Read the model definition and answer for the solid it produces. Units are mm, in the model's axes. A direction names the side the tool comes from. Give positions to 0.01 mm unless a question says otherwise; leave off trailing zeros. Write each loop counter-clockwise with the first axis right and the second up, starting at its lowest first coordinate (ties: lowest second). Pieces come first, ordered by that corner, then holes. Notation, with made-up numbers: (19, 89.25) - (42, 89.25) arc R28 ccw to (42, 110.25) - close; hole circle Ø8 at (8.5, -35.75). An arc over 180 degrees is marked (long way). Use CSV: the item, a comma, the result in double quotes. Start each with the question number.
from build123d import *

# Parameters (mm, degrees)
SKETCH2_OUTSIDE_W       = 53.436
SKETCH2_OUTSIDE_H       = 53.436
CUT_EXTRUDE1_DEPTH      = 8.5
CHAMFER1_SIZE           = 1.754
SKETCH5_W               = 1.79
SKETCH5_H               = 3.988
CUT_EXTRUDE2_DEPTH      = 19
CUT_EXTRUDE2_DEPTH_BACK = 19
SKETCH6_W               = 1.075
SKETCH6_H               = 5.994
CUT_EXTRUDE3_DEPTH      = 19
CUT_EXTRUDE3_DEPTH_BACK = 19


with BuildPart() as part:
    # Sketch1 → Revolve1 (revolve)
    with BuildSketch(Plane.XY, mode=Mode.PRIVATE) as revolve1_sk:
        Polygon((-17.125, 0), (-17, 0), (-17, -2.75), (0, -2.75), (0, 55.25), (-11.75, 55.25), (-18, 53.575317547), (-18, 49.125), (-16.875, 48), (-16.875, 46.5), (-17.925, 45.45), (-17.925, 7.45), (-17.125, 6.65), align=None)
    revolve(revolve1_sk.sketch.rotate(Axis((0, 0, 0), (0, -1, 0)), 270), axis=Axis((0, 0, 0), (0, -1, 0)))  # turned: the seam where the file's is

    # Sketch2 outside → Cut-Extrude1 (cut)
    with BuildSketch(Plane(origin=(0, 55.25, 0), x_dir=(1, 0, 0), z_dir=(0, 1, 0))):
        Rectangle(SKETCH2_OUTSIDE_W, SKETCH2_OUTSIDE_H)
        Polygon((0, 18.429020593), (-15.96, 9.214510296), (-15.96, -9.214510296), (0, -18.429020593), (15.96, -9.214510296), (15.96, 9.214510296), align=None, mode=Mode.SUBTRACT)
    extrude(amount=-CUT_EXTRUDE1_DEPTH, mode=Mode.SUBTRACT)

    # Sketch4 → Revolve2 (revolve)
    with BuildSketch(Plane.XY, mode=Mode.PRIVATE) as revolve2_sk:
        Polygon((0, 70.25), (-6.25, 70.25), (-6.25, 66.262), (-7.25, 66.262), (-7.25, 60.268), (-7.5, 60.268), (-7.5, 55.25), (0, 55.25), align=None)
    revolve(revolve2_sk.sketch.rotate(Axis((0, 0, 0), (0, 1, 0)), 90), axis=Axis((0, 0, 0), (0, 1, 0)))  # turned: the seam where the file's is

    # Chamfer1
    chamfer1_edges = [part.edges().sort_by_distance(p)[0] for p in [
        (0, 70.25, -6.25),
    ]]
    chamfer(chamfer1_edges, length=CHAMFER1_SIZE)

    # Sketch5 → Cut-Extrude2 (cut, two sides)
    with BuildSketch(Plane.XY) as cut_extrude2_sk:
        with Locations((-6.355, 68.256)):
            Rectangle(SKETCH5_W, SKETCH5_H)
        with Locations((6.355, 68.256)):
            Rectangle(SKETCH5_W, SKETCH5_H)
    extrude(amount=CUT_EXTRUDE2_DEPTH, mode=Mode.SUBTRACT)
    extrude(cut_extrude2_sk.sketch, amount=-CUT_EXTRUDE2_DEPTH_BACK, mode=Mode.SUBTRACT)

    # Sketch6 → Cut-Extrude3 (cut, two sides)
    with BuildSketch(Plane.XY) as cut_extrude3_sk:
        with Locations((-6.9625, 63.265)):
            Rectangle(SKETCH6_W, SKETCH6_H)
        with Locations((6.9625, 63.265)):
            Rectangle(SKETCH6_W, SKETCH6_H)
    extrude(amount=CUT_EXTRUDE3_DEPTH, mode=Mode.SUBTRACT)
    extrude(cut_extrude3_sk.sketch, amount=-CUT_EXTRUDE3_DEPTH_BACK, mode=Mode.SUBTRACT)


solid = part.part
(1) The part is cut by section A-A on y = 9. Write down the section's boundary in (x, z) (3 decimals).
(2) For a pull along Y with two mould halves and no side action, classify faces 1 (the face through (14.963, 48.43, -8.693)), 2 (the face through (-0.11, 63.22, 7.25)), 3 (the face through (-3.647, 55.145, 11.58)) as pulls with the +Y half, pulls with the -Y half, needs draft (parallel to the pull), parting line crosses it, or undercut.
(3) Consider probe 1 along Y at (x, z) = (-6, 2.5); probe 2 along X at (y, z) = (58.5, 0.5); probe 3 along Y at (x, z) = (6.5, 6.5). Determine where each line is inside the solid, lowest interval first.
(4) The part is cut by section B-B on y = 64. Write down the section's boundary in (x, z) (3 decimals), plus the area to 3 significant figures.
(5) Given P1, Ø1.5, axis at y = 45, z = 11, coming from the +X side; P2, Ø8, axis at y = 49, z = 2.5, coming from the +X side; P3, Ø8, axis at x = 8.5, y = 17.5, coming from the -Z side; P4, Ø7, axis at x = 0.5, z = 4.5, coming from the +Y side, each flat-ended and moving along its own axis, determine where each tip first touches the part or whether it passes through.
(6) Which of the six approach directions +Z, -Z, +X, -X, +Y, -Y give full straight-line access (tool end or side, diameter ignored) to faces 4 (the face through (8, 55.25, 0)), 5 (the face through (8.081, 50.488, -13.764)), 6 (the face through (5.46, 68, 0)), 7 (the face through (-6.425, 63, 0))?
Reported:
1,outline,"circle Ø35.85 at (0, 0)"
2,face 1,"undercut"
2,face 2,"needs draft"
2,face 3,"pulls with the +Y half"
3,probe 1,"-2.75 to 66.26"
3,probe 2,"-7.48 to 7.48"
3,probe 3,"-2.75 to 55.25"
4,outline,"(-6.425, -3.359) arc R7.25 ccw to (6.425, -3.359) - (6.425, 3.359) arc R7.25 ccw to (-6.425, 3.359) - close"
4,area,"158 mm²"
5,P1,"x = 14.71"
5,P2,"x = 17.91"
5,P3,"z = -17.35"
5,P4,"y = 70.25"
6,face 4,"+Y"
6,face 5,"-Z, +X, +Y"
6,face 6,"+Z, -Z, +X, +Y"
6,face 7,"+Z, -Z, -X, +Y"
